Here's how the part is built. I have some questions about the finished solid (model axes, mm). Face numbers are marked on the shaded views. A direction names the side the tool comes from. Coordinates: 2 decimals unless noted, no trailing zeros. Write each loop counter-clockwise with the first axis right and the second up, starting at its lowest first coordinate (ties: lowest second). Pieces come first, ordered by that corner, then holes. Notation, with made-up numbers: (12, 32) -> (46, 32) arc R33 cw to (46, 67) -> close; hole circle Ø3 at (-36.75, 27.5). An arc over 180 degrees is marked (long way). Put each result on its own line as item: value. Start each with the question number.
Item 1: For pin 1 (2.5 mm diameter, centred on y = -3, z = 19.5, fed in from +X); pin 2 (4 mm diameter, centred on y = -2, z = 18, fed in from -X); pin 3 (4 mm diameter, centred on y = -5.5, z = -41, fed in from -X), each with a flat end and sliding along its axis, tell me the tip position at first contact or that it passes through.
Item 2: I want a section at B-B, the plane x = -9.5. List the corners of the cut face in (y, z) for me.
Item 3: On a 3-axis mill with a long thin cutter (end or side, diameter ignored), from which of +Z, -Z, +X, -X, +Y, -Y can I reach the whole of each face in a straight line? I mean the marked faces 5, 6, 7, 8 and 9. Say none if no direction works.
Item 4: If we mould it in two halves opening along Z, with no side actions, what happens to the marked faces 1, 2, 3 and 4? For each: released by +Z, released by -Z, zero draft, split by the parting line, or undercut.
Item 5: I need wall thicknesses on line 1 (X direction, y = -3.25, z = 30); line 2 (X direction, y = -2, z = -17); line 3 (X direction, y = -2.5, z = -24). Which ranges of each line are inside material? Lowest first, please. Write a range as [from, to].
Item 6: I want a section at A-A, the plane z = 23. List the corners of the cut face in (x, y) for me.
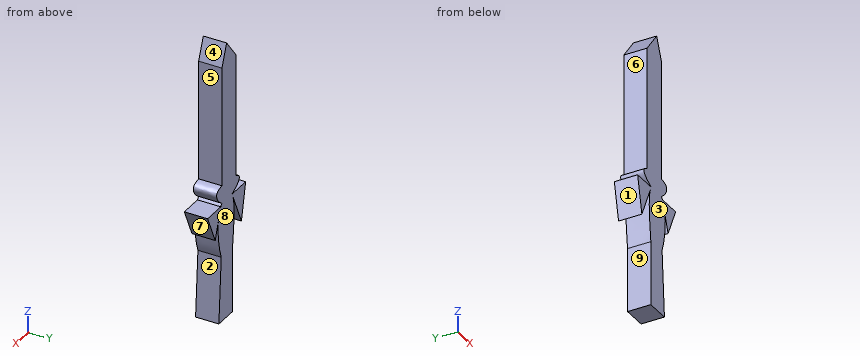
from build123d import *

# Parameters (mm, degrees)
F1_DEPTH = 7.62


with BuildPart() as f1:
    # F0 (on Front) → F1 (new body)
    with BuildSketch(Plane.XZ):
        with BuildLine():
            add(Edge.make_bspline(
                [(-3.6225296477, -15.809470365), (-5.221652466, -20.6566191195), (-3.0213163838, -32.7604657838), (-3.4122510352, -32.7973512532), (-3.3561242744, -32.8900180757)],
                knots=[0.0229994551, 0.0229994551, 0.0229994551, 0.0229994551, 0.2732662158, 0.3066490858, 0.3066490858, 0.3066490858, 0.3066490858], degree=3))
            add(Edge.make_bspline(
                [(-3.3561242744, -32.8900180757), (-3.1358457295, -33.2537039993), (0.4806107603, -36.7303956157), (2.2628287437, -34.532456504), (3.0876353849, -32.3530361056)],
                knots=[0.3066490858, 0.3066490858, 0.3066490858, 0.3066490858, 0.4376655552, 0.570837215, 0.570837215, 0.570837215, 0.570837215], degree=3))
            add(Edge.make_bspline(
                [(3.0876353849, -32.3530361056), (4.2694508133, -29.2302767542), (5.3002211715, -23.9077265842), (4.7680724157, -19.67944375)],
                knots=[0.570837215, 0.570837215, 0.570837215, 0.570837215, 0.7616508122, 0.7616508122, 0.7616508122, 0.7616508122], degree=3))
            Line((4.7680724157, -19.67944375), (3.3561252058, -15.4381711036))
            add(Edge.make_bspline(
                [(3.3561252058, -15.4381711036), (3.1559817041, -15.1441789227), (2.9338306018, -14.8749349929), (2.6951951163, -14.6327009425)],
                knots=[0.8358226137, 0.8358226137, 0.8358226137, 0.8358226137, 0.8553020379, 0.8553020379, 0.8553020379, 0.8553020379], degree=3))
            add(Edge.make_bspline(
                [(2.6951951163, -14.6327009425), (0.8124363798, -15.8162346158), (-0.8659672448, -15.5991068238), (-3.0876344535, -14.6327009425)],
                knots=[0.774708827, 0.774708827, 0.774708827, 0.774708827, 1, 1, 1, 1], degree=3))
            Line((-3.0876344535, -14.6327009425), (-3.6225296477, -15.809470365))
        make_face()
        with BuildLine():
            add(Edge.make_bspline(
                [(-3.3561242744, -32.8900180757), (-3.1358457295, -33.2537039993), (0.4806107603, -36.7303956157), (2.2628287437, -34.532456504), (3.0876353849, -32.3530361056)],
                knots=[0.3066490858, 0.3066490858, 0.3066490858, 0.3066490858, 0.4376655552, 0.570837215, 0.570837215, 0.570837215, 0.570837215], degree=3))
            Line((-3.3561242744, -32.8900180757), (-3.3561242744, -53.8322329521))
            Line((-3.3561242744, -53.8322329521), (4.4300844893, -53.8322329521))
            Line((4.4300844893, -53.8322329521), (3.0876353849, -32.3530361056))
        make_face()
        with BuildLine():
            Line((-8.4574334323, -26.4462586492), (-3.6225296477, -15.809470365))
            add(Edge.make_bspline(
                [(-3.0876344535, -14.6327009425), (-3.2987101155, -14.9678229002), (-3.4755706454, -15.3640185604), (-3.6225296477, -15.809470365)],
                knots=[0, 0, 0, 0, 0.0229994551, 0.0229994551, 0.0229994551, 0.0229994551], degree=3))
            Line((-3.0876344535, -14.6327009425), (-10.8738420531, -14.6327009425))
            Line((-10.8738420531, -14.6327009425), (-8.4574334323, -26.4462586492))
        make_face()
        with BuildLine():
            add(Edge.make_bspline(
                [(-3.0876344535, -14.6327009425), (-3.2987101155, -14.9678229002), (-3.4755706454, -15.3640185604), (-3.6225296477, -15.809470365)],
                knots=[0, 0, 0, 0, 0.0229994551, 0.0229994551, 0.0229994551, 0.0229994551], degree=3))
            Line((-3.6225296477, -15.809470365), (-3.0876344535, -14.6327009425))
        make_face()
        with BuildLine():
            Line((3.3561252058, -15.4381711036), (4.7680724157, -19.67944375))
            add(Edge.make_bspline(
                [(4.7680724157, -19.67944375), (4.5612190651, -18.0358535661), (4.1182115982, -16.5576051031), (3.3561252058, -15.4381711036)],
                knots=[0.7616508122, 0.7616508122, 0.7616508122, 0.7616508122, 0.8358226137, 0.8358226137, 0.8358226137, 0.8358226137], degree=3))
        make_face()
        with BuildLine():
            add(Edge.make_bspline(
                [(4.7680724157, -19.67944375), (4.5612190651, -18.0358535661), (4.1182115982, -16.5576051031), (3.3561252058, -15.4381711036)],
                knots=[0.7616508122, 0.7616508122, 0.7616508122, 0.7616508122, 0.8358226137, 0.8358226137, 0.8358226137, 0.8358226137], degree=3))
            Line((4.7680724157, -19.67944375), (6.5245554865, -24.9556492271))
            Line((6.5245554865, -24.9556492271), (10.8506819233, -15.4381711036))
            Line((10.8506819233, -15.4381711036), (3.3561252058, -15.4381711036))
        make_face()
        with BuildLine():
            add(Edge.make_bspline(
                [(-3.0876344535, -14.6327009425), (-5.2768470806, -13.6804125214), (-8.8119414144, -11.4945501592), (-6.2753688181, -10.0010317936), (-5.4893235481, -9.7083225846)],
                knots=[0, 0, 0, 0, 0.2220000722, 0.288874532, 0.288874532, 0.288874532, 0.288874532], degree=3))
            add(Edge.make_bspline(
                [(2.6951951163, -14.6327009425), (0.9225519342, -12.8333267335), (-1.7596804655, -12.5243264561), (-3.0876344535, -14.6327009425)],
                knots=[0.8553020379, 0.8553020379, 0.8553020379, 0.8553020379, 1, 1, 1, 1], degree=3))
            add(Edge.make_bspline(
                [(2.6801864152, -8.8047577827), (3.8798069065, -8.9398774496), (7.3812464459, -9.985272411), (4.5458992243, -13.4693173455), (2.6951951163, -14.6327009425)],
                knots=[0.4681393873, 0.4681393873, 0.4681393873, 0.4681393873, 0.5532533153, 0.774708827, 0.774708827, 0.774708827, 0.774708827], degree=3))
            add(Edge.make_bspline(
                [(-5.4893235481, -9.7083225846), (-3.3822367481, -8.9236811218), (0.1535753352, -8.5201720741), (2.6801864152, -8.8047577827)],
                knots=[0.288874532, 0.288874532, 0.288874532, 0.288874532, 0.4681393873, 0.4681393873, 0.4681393873, 0.4681393873], degree=3))
        make_face()
        with BuildLine():
            add(Edge.make_bspline(
                [(2.6951951163, -14.6327009425), (0.9225519342, -12.8333267335), (-1.7596804655, -12.5243264561), (-3.0876344535, -14.6327009425)],
                knots=[0.8553020379, 0.8553020379, 0.8553020379, 0.8553020379, 1, 1, 1, 1], degree=3))
            add(Edge.make_bspline(
                [(2.6951951163, -14.6327009425), (0.8124363798, -15.8162346158), (-0.8659672448, -15.5991068238), (-3.0876344535, -14.6327009425)],
                knots=[0.774708827, 0.774708827, 0.774708827, 0.774708827, 1, 1, 1, 1], degree=3))
        make_face()
        with BuildLine():
            Line((-5.4893235481, 30.3271058947), (-5.4893235481, -9.7083225846))
            add(Edge.make_bspline(
                [(-5.4893235481, -9.7083225846), (-3.3822367481, -8.9236811218), (0.1535753352, -8.5201720741), (2.6801864152, -8.8047577827)],
                knots=[0.288874532, 0.288874532, 0.288874532, 0.288874532, 0.4681393873, 0.4681393873, 0.4681393873, 0.4681393873], degree=3))
            Line((2.6801864152, -8.8047577827), (2.6801864152, 30.3271058947))
            Line((2.6801864152, 30.3271058947), (0, 37.272028625))
            Line((0, 37.272028625), (-5.4893235481, 30.3271058947))
        make_face()
    extrude(amount=F1_DEPTH)


solid = f1.part
Calculated:
1. pin 1: stops at x = 2.68
1. pin 2: stops at x = -5.49
1. pin 3: stops at x = -3.36
2. outline: (-7.62, -21.35) -> (0, -21.35) -> (0, -14.63) -> (-7.62, -14.63) -> close
3. face 5: +Z, +X, +Y, -Y
3. face 6: +Z, -X, +Y, -Y
3. face 7: -Z, +X, +Y, -Y
3. face 8: +Z, -Z, +X, -X, +Y
3. face 9: -Z, -X, +Y, -Y
4. face 1: released by -Z
4. face 2: undercut
4. face 3: zero draft
4. face 4: released by +Z
5. line 1: x = [-5.49, 2.68]
5. line 2: x = [-10.39, -4.16], [-3.93, 10.14]
5. line 3: x = [-8.96, -7.35], [-4.17, 4.84], [6.21, 6.96]
6. outline: (-5.49, -7.62) -> (2.68, -7.62) -> (2.68, 0) -> (-5.49, 0) -> close
